Build history of the part. All positions in model axes, mm. A direction names the side the tool comes from. Round coordinates to 2 decimals unless told otherwise and drop trailing zeros. Write each loop counter-clockwise with the first axis right and the second up, starting at its lowest first coordinate (ties: lowest second). Pieces come first, ordered by that corner, then holes.
1) Saw through at C-C (z = 12.7). Write the cut outline in (x, y) (3 decimals).
2) Pull direction Z, two halves, no side cores. Call faces 1 (the flat face through (3, -14, 0)), 2 (the flat face through (50.8, -2, 25)), 3 (the cylindrical face through (12, -1.6, 34.8)): +Z half, -Z half, draft (parallel to the pull), parting line (faces both ways), or undercut.
3) Flat gauge pins, fed straight in: pin 1 (5.5 mm diameter, centred on y = -38.1, z = 38.1, fed in from +X); pin 2 (14.5 mm diameter, centred on x = 24, z = 21.5, fed in from -Y) (3 decimals); pin 3 (1 mm diameter, centred on y = -32, z = 20, fed in from +X) (3 decimals). Where does each tip first touch, or does it go through?
4) Wall check: probe 1 along Z at (x, y) = (12.7, -1.25); probe 2 along Z at (x, y) = (38, -1); probe 3 along Y at (x, z) = (1, 38). Give the ranges that are in metal, low to high.
5) Saw through at A-A (x = 38.1). Write the cut outline in (y, z) (3 decimals), plus the area to 3 significant figures.
6) Saw through at D-D (z = 47.5). Write the cut outline in (x, y) (3 decimals).
7) Which spindle directions (+Z, -Z, +X, -X, +Y, -Y) get a long thin tool onto all of the face, cutting with end or side? Do faces 4 (the cylindrical face through (1.61, -35.256, 36.286)), 5 (the flat face through (27, -3.175, 25)). Say none if no direction does.
8) Saw through at B-B (y = -12.7). Write the cut outline in (x, z) (3 decimals), plus the area to 3 significant figures.
Autodesk Inventor part; units mm, degrees
ref_plane "YZ Plane" through (0, 0, 0) normal (1, 0, 0) x (0, 1, 0)
ref_plane "XZ Plane" through (0, 0, 0) normal (0, 1, 0) x (-1, 0, 0)
ref_plane "XY Plane" through (0, 0, 0) normal (0, 0, 1) x (1, 0, 0)
sketch "Sketch1" plane through (0, 0, 0) normal (0, 0, 1) x (1, 0, 0)
  line L0 (0, 0) -> (50.8, 0)
  line L1 (50.8, 0) -> (50.8, -3.175)
  line L2 (50.8, -3.175) -> (3.175, -3.175)
  line L3 (3.175, -3.175) -> (3.175, -50.8)
  line L4 (3.175, -50.8) -> (0, -50.8)
  line L5 (0, -50.8) -> (0, 0)
  dimension "d0" = 50.8
  dimension "d1" = 3.175
  dimension "d2" = 47.625
  dimension "d3" = 47.625
extrude "Extrusion1" add sketch "Sketch1" along normal blind 50.8
sketch "Sketch2" plane through (3.175, -50.8, 0) normal (1, 0, 0) x (0, 0, -1)
  line L0 (0, 50.8) -> (-50.8, 50.8)
  circle A0 centre (-38.1, 12.7) radius 3.3734
  circle A1 centre (-12.7, 38.1) radius 3.3734
  line L1 (0, 47.625) -> (0, 0)
  point P0 (-50.8, 0)
  dimension "d13" = 38.1
  dimension "d14" = 25.4
  dimension "d15" = 12.7
  dimension "d20" = 6.7469
  dimension "d21" = 6.7469
  dimension "d30" = 38.1
sketch "Sketch3" plane through (3.175, -3.175, 0) normal (0, -1, 0) x (1, 0, 0)
  circle A0 centre (9.525, 38.1) radius 3.3734
  circle A1 centre (34.925, 12.7) radius 3.3734
  line L0 (47.625, 0) -> (0, 0)
  line L1 (47.625, 0) -> (47.625, 50.8)
  line L2 (0, 50.8) -> (47.625, 50.8)
  line L3 (0, 0) -> (0, 50.8)
  point P0 (-3.175, 0)
  dimension "d22" = 6.7469
  dimension "d23" = 6.7469
  dimension "d24" = 12.7
  dimension "d25" = 12.7
  dimension "d26" = 12.7
  dimension "d27" = 9.525
extrude "Extrusion4" cut sketch "Sketch3" against normal blind 3.175 contours A0 | A1
extrude "Extrusion5" cut sketch "Sketch2" against normal blind 3.175
properties part number "angle gusset" material "Aluminum 6061"
Evaluation:
1. outline: (0, -50.8) - (3.175, -50.8) - (3.175, -16.073) - (0, -16.073) - close; (0, -9.327) - (3.175, -9.327) - (3.175, -3.175) - (34.727, -3.175) - (34.727, 0) - (0, 0) - close; (41.473, -3.175) - (50.8, -3.175) - (50.8, 0) - (41.473, 0) - close
2. face 1: -Z half
2. face 2: draft
2. face 3: undercut
3. pin 1: passes through
3. pin 2: stops at y = -3.175
3. pin 3: stops at x = 3.175
4. probe 1: z = 0 to 34.73, 41.47 to 50.8
4. probe 2: z = 0 to 9.33, 16.07 to 50.8
4. probe 3: y = -50.8 to -41.47, -34.73 to 0
5. outline: (-3.175, 0) - (0, 0) - (0, 9.327) - (-3.175, 9.327) - close; (-3.175, 16.073) - (0, 16.073) - (0, 50.8) - (-3.175, 50.8) - close
5. area: 140 mm2
6. outline: (0, -50.8) - (3.175, -50.8) - (3.175, -3.175) - (50.8, -3.175) - (50.8, 0) - (0, 0) - close
7. face 4: +X, -X
7. face 5: +Z, -Z, +X, -Y
8. outline: (0, 0) - (3.175, 0) - (3.175, 9.327) - (0, 9.327) - close; (0, 16.073) - (3.175, 16.073) - (3.175, 50.8) - (0, 50.8) - close
8. area: 140 mm2
